Geometry: see drawing. Coordinates: mm, zero at the bounding-box minimum. A direction names the side the tool comes from. Coordinates: 2 decimals unless noted, no trailing zeros. Order: outer loops, then holes, each group sorted by start corner. A loop starts at its lowest first (then second) coordinate and runs counter-clockwise, first axis right, second up. Notation, with made-up numbers: M 37,71 L 94,71 A17 ccw 94,94 Z; hole C 48.5,-8.75 d5. An arc over 180 degrees is marked long. Answer in a Markdown table with one row per item.
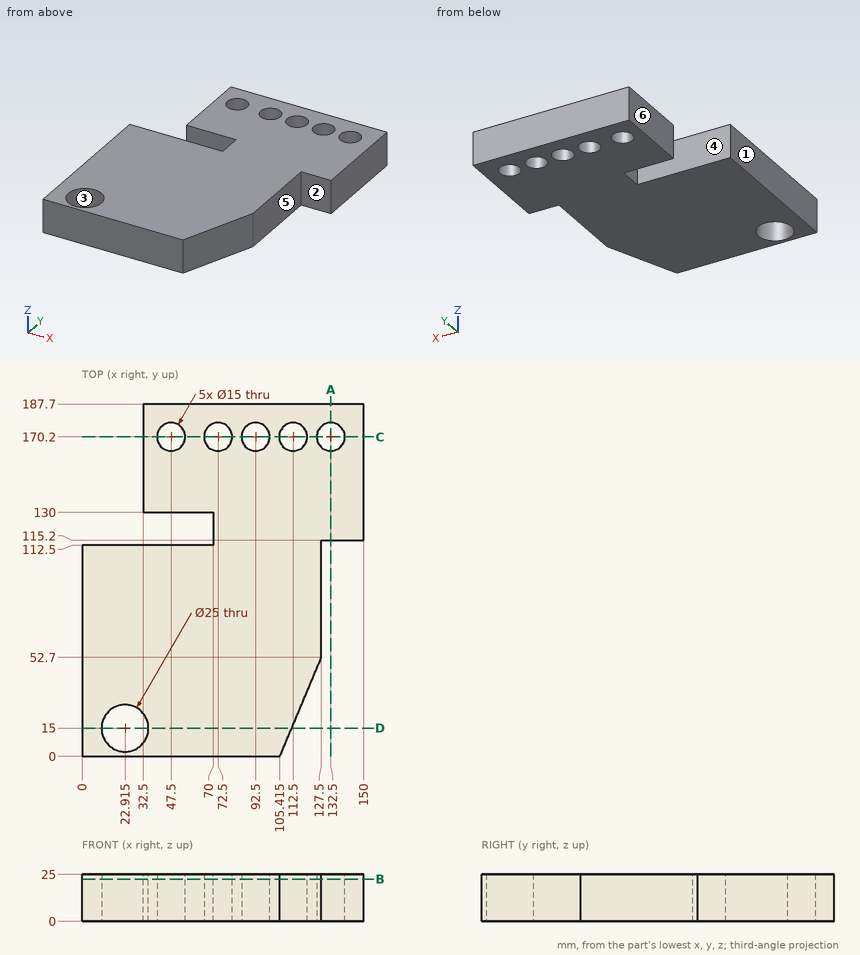
1) Reachability of the marked faces 4, 5 and 6 from +Z, -Z, +X, -X, +Y, -Y: full face, straight path, thin tool, end or side. Return the list, or none.
Resolved:
| item | result |
|---|---|
| face 4 | +Z, -Z, -X |
| face 5 | +Z, -Z, +X, -Y |
| face 6 | +Z, -Z, -X, +Y |
2) Contact query for flat-ended pins moving along their axis: pin 1 (20 mm diameter, centred on x = 22.92, y = 15, fed in from -Z) (3 decimals); pin 2 (5 mm diameter, centred on x = 19.5, z = 18, fed in from +Y); pin 3 (5 mm diameter, centred on y = 129, z = 19.5, fed in from -X); pin 4 (3 mm diameter, centred on y = 52.5, z = 17, fed in from +X). Output: stop coordinate, or through.
Resolved:
| item | result |
|---|---|
| pin 1 | passes through |
| pin 2 | stops at y = 112.5 |
| pin 3 | stops at x = 32.5 |
| pin 4 | stops at x = 127.5 |
3) Cut plane D-D, the plane y = 15. Output: boundary loops of the cut face in (x, z) (1 decimal), and give its area (3 significant figures).
Resolved:
| item | result |
|---|---|
| outline | M 0,0 L 10.4,0 L 10.4,25 L 0,25 Z; M 35.4,0 L 111.7,0 L 111.7,25 L 35.4,25 Z |
| area | 2,170 mm2 |
4) Cut plane A-A, the plane x = 132.5. Output: boundary loops of the cut face in (y, z), and give its area (3 significant figures).
Resolved:
| item | result |
|---|---|
| outline | M 115.2,0 L 162.7,0 L 162.7,25 L 115.2,25 Z; M 177.7,0 L 187.7,0 L 187.7,25 L 177.7,25 Z |
| area | 1,440 mm2 |
5) Mould query, pull axis Y, two halves, no side actions, for the marked faces 1, 2 and 3. Classes: +Y half, -Y half, draft (parallel to the pull), parting line (faces both ways), or undercut.
Resolved:
| item | result |
|---|---|
| face 1 | draft |
| face 2 | -Y half |
| face 3 | undercut |
6) Material intervals for probe 1 along X at (y, z) = (171, 19.75); probe 2 along Y at (x, z) = (56, 23.5); probe 3 along Y at (x, z) = (132, 22.5), sorted ascending.
Resolved:
| item | result |
|---|---|
| probe 1 | x = 32.5 to 40.04, 54.96 to 65.04, 79.96 to 85.04, 99.96 to 105.04, 119.96 to 125.04, 139.96 to 150 |
| probe 2 | y = 0 to 112.5, 130 to 187.7 |
| probe 3 | y = 115.2 to 162.72, 177.68 to 187.7 |
7) Cut plane B-B, the plane z = 22.5. Output: boundary loops of the cut face in (x, y) (1 decimal), and give its area (3 significant figures).
Resolved:
| item | result |
|---|---|
| outline | M 0,0 L 105.4,0 L 127.5,52.7 L 127.5,115.2 L 150,115.2 L 150,187.7 L 32.5,187.7 L 32.5,130 L 70,130 L 70,112.5 L 0,112.5 Z; hole C 22.9,15 d25; hole C 47.5,170.2 d15; hole C 72.5,170.2 d15; hole C 92.5,170.2 d15; hole C 112.5,170.2 d15; hole C 132.5,170.2 d15 |
| area | 20,500 mm2 |
8) Cut plane C-C, the plane y = 170.2. Output: boundary loops of the cut face in (x, z).
Resolved:
| item | result |
|---|---|
| outline | M 32.5,0 L 40,0 L 40,25 L 32.5,25 Z; M 55,0 L 65,0 L 65,25 L 55,25 Z; M 80,0 L 85,0 L 85,25 L 80,25 Z; M 100,0 L 105,0 L 105,25 L 100,25 Z; M 120,0 L 125,0 L 125,25 L 120,25 Z; M 140,0 L 150,0 L 150,25 L 140,25 Z |
